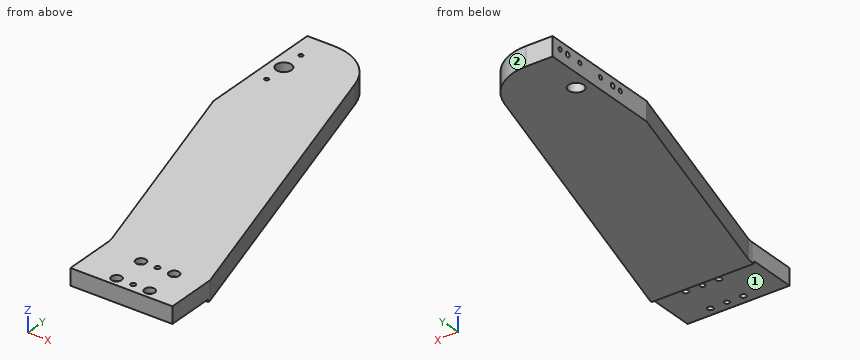
from build123d import *

# Parameters (mm, degrees)
SALIENTE_EXTRUIR1_DEPTH                              = 15
CROQUIS2_R                                           = 6
CORTAR_EXTRUIR1_DEPTH                                = 16
PERFORADOR_PARA_ROSCAR_PARA_MACHO_DE_ROS_D           = 3.3
PERFORADOR_PARA_ROSCAR_PARA_MACHO_DE_ROS_DEPTH       = 7
PERFORADOR_PARA_ROSCAR_PARA_MACHO_DE_ROS_TIP         = 0.991420021
CROQUIS9_W                                           = 80
CROQUIS9_H                                           = 38
CORTAR_EXTRUIR2_DEPTH                                = 2
TALADRO_ROSCADO_M41_D                                = 3.3
TALADRO_ROSCADO_M41_DEPTH                            = 15
TALADRO_ROSCADO_M41_TIP                              = 0.991420021
TALADROS_DE_ESPIGA_DE_4_0MM1_D                       = 4
TALADROS_DE_ESPIGA_DE_4_0MM1_DEPTH                   = 17
TALADROS_DE_ESPIGA_DE_4_0MM1_TIP                     = 1.201721238
TALADROS_DE_ESPIGA_DE_4_0MM3_D                       = 4
REFRENTADO_PARA_TORNILLO_CON_CABEZA_HUEC_D           = 4.5
REFRENTADO_PARA_TORNILLO_CON_CABEZA_HUEC_CBORE_D     = 8
REFRENTADO_PARA_TORNILLO_CON_CABEZA_HUEC_CBORE_DEPTH = 4.4


with BuildPart() as part:
    # Croquis1 → Saliente-Extruir1 (new body)
    with BuildSketch(Plane.XY):
        with BuildLine():
            Line((80, 0), (80, 40))
            Line((80, 40), (9.228509485, 290.860669242))
            ThreePointArc((9.228509485, 290.860669242), (-5.12786552, 311.893782856), (-29.268839302, 320))
            Line((-29.268839302, 320), (-50, 320))
            Line((-50, 320), (-50, 220))
            Line((-50, 220), (-0.751325607, 45.430334621))
            ThreePointArc((-0.751325607, 45.430334621), (-0.1887218, 42.741031935), (0, 40))
            Line((0, 40), (0, 0))
            Line((0, 0), (80, 0))
        make_face()
    extrude(amount=SALIENTE_EXTRUIR1_DEPTH)

    # Croquis2 → Cortar-Extruir1 (cut, through all)
    with BuildSketch(Plane(origin=(0, 0, 0), x_dir=(-1, 0, 0), z_dir=(0, 0, -1))):
        with Locations((39, 280)):
            Circle(CROQUIS2_R)
    extrude(amount=-CORTAR_EXTRUIR1_DEPTH, mode=Mode.SUBTRACT)

    # Perforador para roscar para macho de roscar para M44
    with Locations(Plane.XY.offset(15)):
        with Locations((-39, 298.25), (-39, 261.75)):
            Hole(PERFORADOR_PARA_ROSCAR_PARA_MACHO_DE_ROS_D / 2, depth=PERFORADOR_PARA_ROSCAR_PARA_MACHO_DE_ROS_DEPTH)
            with Locations((0, 0, -(PERFORADOR_PARA_ROSCAR_PARA_MACHO_DE_ROS_DEPTH + PERFORADOR_PARA_ROSCAR_PARA_MACHO_DE_ROS_TIP / 2))):  # 118° drill point
                Cone(0, PERFORADOR_PARA_ROSCAR_PARA_MACHO_DE_ROS_D / 2, PERFORADOR_PARA_ROSCAR_PARA_MACHO_DE_ROS_TIP, mode=Mode.SUBTRACT)

    # Croquis9 → Cortar-Extruir2 (cut)
    with BuildSketch(Plane(origin=(0, 0, 0), x_dir=(-1, 0, 0), z_dir=(0, 0, -1))):
        with Locations((-40, 19)):
            Rectangle(CROQUIS9_W, CROQUIS9_H)
    extrude(amount=-CORTAR_EXTRUIR2_DEPTH, mode=Mode.SUBTRACT)

    # Taladro roscado M41
    with Locations(Plane.ZY.offset(50)):
        with Locations((9, 312), (9, 248), (9, 291), (9, 269)):
            Hole(TALADRO_ROSCADO_M41_D / 2, depth=TALADRO_ROSCADO_M41_DEPTH)
            with Locations((0, 0, -(TALADRO_ROSCADO_M41_DEPTH + TALADRO_ROSCADO_M41_TIP / 2))):  # 118° drill point
                Cone(0, TALADRO_ROSCADO_M41_D / 2, TALADRO_ROSCADO_M41_TIP, mode=Mode.SUBTRACT)

    # Taladros de espiga de Ø4.0mm1
    with Locations(Plane.ZY.offset(50)):
        with Locations((9, 304), (9, 256)):
            Hole(TALADROS_DE_ESPIGA_DE_4_0MM1_D / 2, depth=TALADROS_DE_ESPIGA_DE_4_0MM1_DEPTH)
            with Locations((0, 0, -(TALADROS_DE_ESPIGA_DE_4_0MM1_DEPTH + TALADROS_DE_ESPIGA_DE_4_0MM1_TIP / 2))):  # 118° drill point
                Cone(0, TALADROS_DE_ESPIGA_DE_4_0MM1_D / 2, TALADROS_DE_ESPIGA_DE_4_0MM1_TIP, mode=Mode.SUBTRACT)

    # Taladros de espiga de Ø4.0mm3 (through all)
    with Locations(Plane.XY.offset(15)):
        with Locations((44, 33), (44, 7)):
            Hole(TALADROS_DE_ESPIGA_DE_4_0MM3_D / 2)

    # Refrentado para tornillo con cabeza hueca de M41 (through all)
    with Locations(Plane.XY.offset(15)):
        with Locations((57, 33), (31, 7), (31, 33), (57, 7)):
            CounterBoreHole(REFRENTADO_PARA_TORNILLO_CON_CABEZA_HUEC_D / 2, REFRENTADO_PARA_TORNILLO_CON_CABEZA_HUEC_CBORE_D / 2, REFRENTADO_PARA_TORNILLO_CON_CABEZA_HUEC_CBORE_DEPTH)


solid = part.part
Can you work these out from the model? Positions are in its coordinate system, mm. Face numbers are marked on the shaded views. A direction names the side the tool comes from. Give positions to 0.01 mm unless a question says otherwise; leave off trailing zeros. Write each loop counter-clockwise with the first axis right and the second up, starting at its lowest first coordinate (ties: lowest second). Pieces come first, ordered by that corner, then holes. Notation, with made-up numbers: M 29,51.25 L 58,51.25 A19 cw 58,67.25 Z; hole C 56,-13.5 d8. An arc over 180 degrees is marked long. Answer in a Markdown table with one row per item. Add a question column.
Item 1: Imagine slicing it at B-B, the plane x = -13. Write out the boundary of the cut face in (y, z), plus the area to 3 significant figures.
Item 2: Imagine slicing it at C-C, the plane y = 137. Write out the boundary of the cut face in (x, z), plus the area to 3 significant figures.
Item 3: Please list where these lines run through material, in increasing order: L1, parallel to Z at x = -42.75, y = 256; L2, parallel to Z at x = 45, y = 26; L3, parallel to X at y = 261.75, z = 11.5.
Item 4: On a 3-axis mill with a long thin cutter (end or side, diameter ignored), from which of +Z, -Z, +X, -X, +Y, -Y can I reach the whole of each face in a straight line? I mean the marked faces 1 and 2. Say none if no direction works.
Item 5: Imagine slicing it at A-A, the plane y = 280. Write out the boundary of the cut face in (x, z).
Item 6: For pin 1 Ø2.5 at (y, z) = (291, 9) entering from -X; pin 2 Ø5 at (x, y) = (31, 7) entering from -Z; pin 3 Ø3.5 at (y, z) = (304, 9) entering from +X, each with a flat end and sliding along its axis, tell me the tip position at first contact or that it passes through.
Evaluation:
| question | item | result |
|---|---|---|
| 1 | outline | M 88.85,0 L 316.54,0 L 316.54,15 L 88.85,15 Z |
| 1 | area | 3,420 mm² |
| 2 | outline | M -26.58,0 L 52.63,0 L 52.63,15 L -26.58,15 Z |
| 2 | area | 1,190 mm² |
| 3 | L1 | z = 0 to 7, 11 to 15 |
| 3 | L2 | z = 2 to 15 |
| 3 | L3 | x = -50 to -40.65, -37.35 to 17.44 |
| 4 | face 1 | -Z, +X, -X, -Y |
| 4 | face 2 | +Z, -Z, +X, +Y |
| 5 | outline | M -50,0 L -45,0 L -45,15 L -50,15 Z; M -33,0 L 12.29,0 L 12.29,15 L -33,15 Z |
| 6 | pin 1 | stops at x = -34.76 |
| 6 | pin 2 | stops at z = 2 |
| 6 | pin 3 | stops at x = 3.97 |
